For this review, take the finished solid that the model builds, in its own axes (mm). Face numbers are marked on the shaded views. A direction names the side the tool comes from. Give positions to 0.01 mm unless a question says otherwise; leave off trailing zeros. Order: outer loops, then holes, each group sorted by start corner. A loop starts at its lowest first (then second) coordinate and runs counter-clockwise, first axis right, second up. Notation, with made-up numbers: (-1, 58) -> (11, 58) arc R11 ccw to (11, 76) -> close; hole circle Ø5 at (-24, -8.75). An arc over 180 degrees is marked (long way). Return JSON: item names as keys, results as strings. Group by question number.
1) Add section A-A (x = 90). Give the boundary of the cut face in (y, z).
2) To check wall thickness, follow line 1 along X through (y, z) = (-42.25, 35); line 2 along Y through (x, z) = (39, 24.5); line 3 along X through (y, z) = (-11, 39). State the ranges of each line that lie inside material, in increasing order.
3) Add section D-D (y = -33.5). Give the boundary of the cut face in (x, z), then the cut area to 3 significant figures.
4) Insertion check: P1, Ø4, axis at y = -13.5, z = 40, coming from the -X side; P2, Ø10, axis at x = 68, y = -20.5, coming from the -Z side; P3, Ø3, axis at x = 7, z = 8, coming from the +Y side; P4, Ø4, axis at x = 28.5, z = 34, coming from the +Y side. Each pin has a flat end and moves straight along its axis. Give the tip position at first contact, or say it passes through.
5) For the marked faces 4, 5 and 6, list the 3-axis set-ups (+Z, -Z, +X, -X, +Y, -Y) from which the entire face can be reached by the end or side of a thin tool; tool diameter is ignored.
6) Add section B-B (y = -20). Give the boundary of the cut face in (x, z), then the cut area to 3 significant figures.
7) Add section C-C (z = 54). Give the boundary of the cut face in (x, y).
8) The part is to be moulded in two halves that separate along X. For the marked faces 1, 2 and 3, say which applies: released by +X, released by -X, zero draft, split by the parting line, or undercut.
from build123d import *

# Parameters (mm, degrees)
F0_W      = 100
F0_H      = 63
F1_DEPTH  = 50
F3_DEPTH  = 6
F4_DEPTH  = 50
F5_DEPTH  = 50
F2_R      = 10
F2_R_2    = 5
F6_DEPTH  = 8
F2_R_3    = 25
F7_DEPTH  = 13
F8_W      = 10
F8_H      = 12
F9_DEPTH  = 63
F10_W     = 40
F10_H     = 12
F11_DEPTH = 63
F12_R     = 5
F13_DEPTH = 50
F15_DEPTH = 50
F16_DEPTH = 42
F17_DEPTH = 42
F18_W     = 30
F18_H     = 8
F19_DEPTH = 11.4
F21_DEPTH = 100
F22_R     = 5
F23_DEPTH = 63


with BuildPart() as f1:
    # F0 (on Front) → F1 (new body)
    with BuildSketch(Plane.XZ):
        with Locations((50, 31.5)):
            Rectangle(F0_W, F0_H)
    extrude(amount=F1_DEPTH)

    # F2 (on face) → F3 (cut)
    with BuildSketch(Plane.XZ.offset(50)):
        with BuildLine():
            ThreePointArc((80, 35), (85.8578643763, 20.8578643763), (100, 15))
            Line((100, 15), (100, 48))
            Line((100, 48), (80, 48))
            Line((80, 48), (80, 35))
        make_face()
    extrude(amount=-F3_DEPTH, mode=Mode.SUBTRACT)

    # F2 (on face) → F4 (cut)
    with BuildSketch(Plane.XZ.offset(50)):
        Polygon((100, 63), (60, 63), (60, 48), (80, 48), (100, 48), align=None)
    extrude(amount=-F4_DEPTH, mode=Mode.SUBTRACT)

    # F2 (on face) → F5 (cut)
    with BuildSketch(Plane.XZ.offset(50)):
        with BuildLine():
            Line((75.1384166813, 5.7840544194), (59.246857771, 0))
            Line((59.246857771, 0), (97.253292799, 0))
            Line((97.253292799, 0), (96.1209551715, 1.1323376275))
            ThreePointArc((96.1209551715, 1.1323376275), (86.3076118266, 6.5161221461), (75.1384166813, 5.7840544194))
        make_face()
    extrude(amount=-F5_DEPTH, mode=Mode.SUBTRACT)

    # F2 (on face) → F6 (cut)
    with BuildSketch(Plane.XZ.offset(50)):
        with Locations((30, 35)):
            Circle(F2_R)
        with Locations((30, 35)):
            Circle(F2_R_2, mode=Mode.SUBTRACT)
    extrude(amount=-F6_DEPTH, mode=Mode.SUBTRACT)

    # F2 (on face) → F7 (cut)
    with BuildSketch(Plane.XZ.offset(50)):
        with Locations((30, 35)):
            Circle(F2_R_3)
        with Locations((30, 35)):
            Circle(F2_R, mode=Mode.SUBTRACT)
    extrude(amount=-F7_DEPTH, mode=Mode.SUBTRACT)

    # F8 (on face) → F9 (cut)
    with BuildSketch(Plane.XY.offset(63)):
        with Locations((55, -6)):
            Rectangle(F8_W, F8_H)
    extrude(amount=-F9_DEPTH, mode=Mode.SUBTRACT)

    # F10 (on face) → F11 (cut)
    with BuildSketch(Plane.XY.offset(48)):
        with Locations((80, -6)):
            Rectangle(F10_W, F10_H)
    extrude(amount=-F11_DEPTH, mode=Mode.SUBTRACT)

    # F12 (on face) → F13 (cut)
    with BuildSketch(Plane.XZ.offset(44)):
        with Locations((90, 38.0427613854)):
            Circle(F12_R)
    extrude(amount=-F13_DEPTH, mode=Mode.SUBTRACT)

    # F14 (on face) → F15 (cut)
    with BuildSketch(Plane(origin=(0, 0, 0), x_dir=(-1, 0, 0), z_dir=(0, 1, 0))):
        with BuildLine():
            Line((0, 10), (0, 60))
            ThreePointArc((0, 60), (-25, 35), (0, 10))
        make_face()
        with BuildLine():
            ThreePointArc((0, 10), (17.6776695297, 17.3223304703), (25, 35))
            ThreePointArc((25, 35), (17.6776695297, 52.6776695297), (0, 60))
            Line((0, 60), (0, 10))
        make_face()
    extrude(amount=-F15_DEPTH, mode=Mode.SUBTRACT)

    # F14 (on face) → F16 (cut)
    with BuildSketch(Plane(origin=(0, 0, 0), x_dir=(-1, 0, 0), z_dir=(0, 1, 0))):
        with BuildLine():
            ThreePointArc((0, 10), (-25, 35), (0, 60))
            Line((0, 60), (0, 63))
            Line((0, 63), (-10.7703296143, 63))
            ThreePointArc((-10.7703296143, 63), (-24.7296369608, 51.9836702684), (-30, 35))
            ThreePointArc((-30, 35), (-21.2132034356, 13.7867965644), (0, 5))
            Line((0, 5), (0, 10))
        make_face()
        with BuildLine():
            ThreePointArc((0, 60), (17.6776695297, 52.6776695297), (25, 35))
            ThreePointArc((25, 35), (17.6776695297, 17.3223304703), (0, 10))
            Line((0, 10), (0, 5))
            ThreePointArc((0, 5), (21.2132034356, 13.7867965644), (30, 35))
            ThreePointArc((30, 35), (16.9836702684, 59.7296369608), (-10.7703296143, 63))
            Line((-10.7703296143, 63), (0, 63))
            Line((0, 63), (0, 60))
        make_face()
    extrude(amount=F16_DEPTH, mode=Mode.SUBTRACT)

    # F14 (on face) → F17 (cut)
    with BuildSketch(Plane(origin=(0, 0, 0), x_dir=(-1, 0, 0), z_dir=(0, 1, 0))):
        with BuildLine():
            ThreePointArc((0, 10), (-25, 35), (0, 60))
            Line((0, 60), (0, 63))
            Line((0, 63), (-10.7703296143, 63))
            ThreePointArc((-10.7703296143, 63), (-24.7296369608, 51.9836702684), (-30, 35))
            ThreePointArc((-30, 35), (-21.2132034356, 13.7867965644), (0, 5))
            Line((0, 5), (0, 10))
        make_face()
        with BuildLine():
            ThreePointArc((0, 60), (17.6776695297, 52.6776695297), (25, 35))
            ThreePointArc((25, 35), (17.6776695297, 17.3223304703), (0, 10))
            Line((0, 10), (0, 5))
            ThreePointArc((0, 5), (21.2132034356, 13.7867965644), (30, 35))
            ThreePointArc((30, 35), (16.9836702684, 59.7296369608), (-10.7703296143, 63))
            Line((-10.7703296143, 63), (0, 63))
            Line((0, 63), (0, 60))
        make_face()
        with BuildLine():
            ThreePointArc((-30, 35), (-24.7296369608, 51.9836702684), (-10.7703296143, 63))
            Line((-10.7703296143, 63), (-30, 63))
            Line((-30, 63), (-30, 35))
        make_face()
    extrude(amount=-F17_DEPTH, mode=Mode.SUBTRACT)

    # F18 (on face) → F19 (cut)
    with BuildSketch(Plane.XY.offset(63)):
        with Locations((15, -46)):
            Rectangle(F18_W, F18_H)
    extrude(amount=-F19_DEPTH, mode=Mode.SUBTRACT)

    # F20 (on face) → F21 (cut)
    with BuildSketch(Plane(origin=(30, 0, 0), x_dir=(0, -1, 0), z_dir=(-1, 0, 0))):
        Polygon((6.5514642168, 63), (0, 63), (0, 45), align=None)
    extrude(amount=-F21_DEPTH, mode=Mode.SUBTRACT)

    # F22 (on face) → F23 (cut)
    with BuildSketch(Plane.XY.offset(63)):
        with Locations((39, -20)):
            Circle(F22_R)
    extrude(amount=-F23_DEPTH, mode=Mode.SUBTRACT)


solid = f1.part
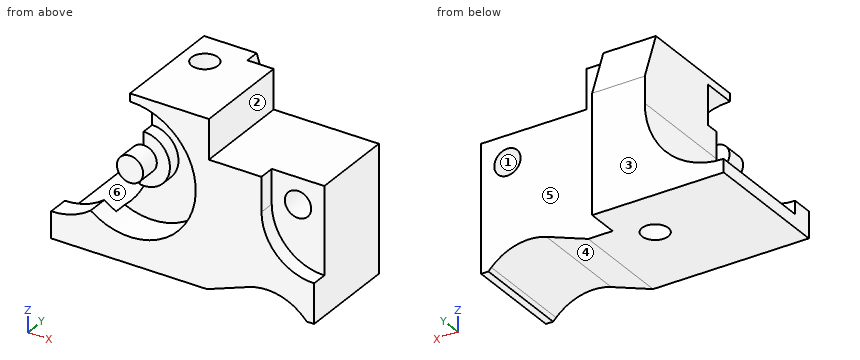
Evaluation:
{
 "1": {"outline": "(-50, 5.31) -> (-12, 5.31) -> (-12, 33.04) -> (-44, 33.04) -> (-44, 17.68) -> (-50, 17.68) -> close; (-44, 43.04) -> (-12, 43.04) -> (-12, 48) -> (-44, 48) -> close"},
 "2": {"line 1": "25 to 35, 55 to 86.03, 93.97 to 100", "line 2": "-37 to -25, -15 to 0", "line 3": "30 to 50"},
 "3": {"outline": "(0, 0) -> (59.25, 0) -> (75.14, 5.78) arc R20 cw to (96.12, 1.13) -> (97.25, 0) -> (100, 0) -> (100, 48) -> (60, 48) -> (60, 63) -> (30, 63) -> (30, 35) arc R30 cw to (0, 5) -> close; hole circle Ø10 at (90, 38.04)", "area": "3,910 mm^2"},
 "4": {"P1": "x = 30", "P2": "z = 1.37", "P3": "y = -42", "P4": "y = 0"},
 "5": {"face 4": "-Z, +Y, -Y", "face 5": "+Z, -Z, +X, +Y", "face 6": "+Z, -X, +Y"},
 "6": {"outline": "(0, 0) -> (34, 0) -> (34, 63) -> (30, 63) -> (30, 35) arc R30 cw to (0, 5) -> close; (44, 0) -> (59.25, 0) -> (75.14, 5.78) arc R20 cw to (96.12, 1.13) -> (97.25, 0) -> (100, 0) -> (100, 48) -> (60, 48) -> (60, 63) -> (44, 63) -> close; hole circle Ø10 at (90, 38.04)", "area": "3,280 mm^2"},
 "7": {"outline": "(30, -37) -> (46.25, -37) -> (46.25, -50) -> (60, -50) -> (60, -12) -> (50, -12) -> (50, -3.28) -> (30, -3.28) -> close; hole circle Ø10 at (39, -20)"},
 "8": {"face 1": "undercut", "face 2": "released by +X", "face 3": "zero draft"}
}
